from build123d import *

# Parameters (mm, degrees)
AUFSATZ_LINEAR_AUSTRAGEN1_DEPTH  = 16.09
WANDUNG2_T                       = -0.6
VERRUNDUNG1_R                    = 2
VERRUNDUNG2_R                    = 2
SKIZZE7_R                        = 2.5
AUFSATZ_LINEAR_AUSTRAGEN4_DEPTH  = 10
FASE3_SIZE                       = 0.5
AUFSATZ_LINEAR_AUSTRAGEN8_DEPTH  = 7.85
SKIZZE14_W                       = 3.695
SKIZZE14_H                       = 14.25
AUFSATZ_LINEAR_AUSTRAGEN9_DEPTH  = 2.94
SKIZZE15_W                       = 14.89
SKIZZE15_H                       = 14.52
AUFSATZ_LINEAR_AUSTRAGEN10_DEPTH = 1.06
SCHNITT_LINEAR_AUSTRAGEN1_REACH  = 12.16
SKIZZE16_W                       = 4.8
SKIZZE16_H                       = 5.3
SKIZZE17_W                       = 14.89
SKIZZE17_H                       = 14.52
AUFSATZ_LINEAR_AUSTRAGEN11_DEPTH = 1.06
SCHNITT_LINEAR_AUSTRAGEN2_REACH  = 12.16
SKIZZE18_W                       = 4.8
SKIZZE18_H                       = 5.3


with BuildPart() as part:
    # Skizze4 → Aufsatz-Linear austragen1 (new body)
    with BuildSketch(Plane.XY):
        Polygon((-6.4, 0), (-20, 14.7), (20, 14.7), (6.4, 0), align=None)
    extrude(amount=AUFSATZ_LINEAR_AUSTRAGEN1_DEPTH)

    # Wandung2
    wandung2_openings = [part.faces().sort_by_distance(p)[0] for p in [
        (0, 14.7, 8.045),
        (0, 0, 8.045),
    ]]
    offset(amount=WANDUNG2_T, openings=wandung2_openings, kind=Kind.INTERSECTION)

    # Verrundung1
    verrundung1_edges = [part.edges().sort_by_distance(p)[0] for p in [
        (12.382602743, 7.35, 15.49),
        (-12.382602743, 7.35, 15.49),
    ]]
    fillet(verrundung1_edges, radius=VERRUNDUNG1_R)

    # Verrundung2
    verrundung2_edges = [part.edges().sort_by_distance(p)[0] for p in [
        (12.382602743, 7.35, 0.6),
        (-12.382602743, 7.35, 0.6),
    ]]
    fillet(verrundung2_edges, radius=VERRUNDUNG2_R)

    # Skizze7 → Aufsatz-Linear austragen4 (add)
    with BuildSketch(Plane(origin=(0, 0, 0), x_dir=(-1, 0, 0), z_dir=(0, 0, -1))):
        with Locations((-14.281252926, 12.2)):
            Circle(SKIZZE7_R)
        with Locations((14.281252926, 12.2)):
            Circle(SKIZZE7_R)
    extrude(amount=AUFSATZ_LINEAR_AUSTRAGEN4_DEPTH)

    # Fase3
    fase3_edges = [part.edges().sort_by_distance(p)[0] for p in [
        (16.781252926, 12.2, -10),
        (-11.781252926, 12.2, -10),
    ]]
    chamfer(fase3_edges, length=FASE3_SIZE)

    # Skizze12 → Aufsatz-Linear austragen8 (add, symmetric)
    with BuildSketch(Plane.XY.offset(8.045)):
        Polygon((6.9, 0.540441176), (6.9, 10), (10.9, 10), (10.9, 4.863970588), align=None)
    aufsatz_linear_austragen8 = extrude(amount=AUFSATZ_LINEAR_AUSTRAGEN8_DEPTH, both=True)

    # Spiegeln6: Aufsatz-Linear austragen8 across plane
    add(aufsatz_linear_austragen8.mirror(Plane(origin=(0, 0, 0), x_dir=(0, 0, 1), z_dir=(1, 0, 0))))

    # Skizze14 → Aufsatz-Linear austragen9 (add)
    with BuildSketch(Plane.ZY.offset(-9.84)):
        with Locations((2.4475, 17.125)):
            Rectangle(SKIZZE14_W, SKIZZE14_H)
        with Locations((13.6425, 17.125)):
            Rectangle(SKIZZE14_W, SKIZZE14_H)
    aufsatz_linear_austragen9 = extrude(amount=AUFSATZ_LINEAR_AUSTRAGEN9_DEPTH)

    # Skizze15 → Aufsatz-Linear austragen10 (add)
    with BuildSketch(Plane(origin=(9.84, 0, 0), x_dir=(0, 0, -1), z_dir=(1, 0, 0))):
        with Locations((-8.045, 16.99)):
            Rectangle(SKIZZE15_W, SKIZZE15_H)
    extrude(amount=AUFSATZ_LINEAR_AUSTRAGEN10_DEPTH)

    # Skizze16 → Schnitt-Linear austragen1 (cut, up to next)
    with BuildSketch(Plane.ZY.offset(-9.84), mode=Mode.PRIVATE) as schnitt_linear_austragen1_sk1:
        with Locations((7.345, 21.6)):
            Rectangle(SKIZZE16_W, SKIZZE16_H)
    schnitt_linear_austragen1_tool1 = extrude(schnitt_linear_austragen1_sk1.sketch, amount=-SCHNITT_LINEAR_AUSTRAGEN1_REACH, mode=Mode.PRIVATE) & part.part
    add(schnitt_linear_austragen1_tool1.solids().sort_by_distance((9.84, 21.6, 7.345))[0], mode=Mode.SUBTRACT)

    # Spiegeln9: Aufsatz-Linear austragen9 across plane
    add(aufsatz_linear_austragen9.mirror(Plane(origin=(0, 0, 0), x_dir=(0, 0, 1), z_dir=(1, 0, 0))))

    # Skizze17 → Aufsatz-Linear austragen11 (add)
    with BuildSketch(Plane.ZY.offset(9.84)):
        with Locations((8.045, 16.99)):
            Rectangle(SKIZZE17_W, SKIZZE17_H)
    extrude(amount=AUFSATZ_LINEAR_AUSTRAGEN11_DEPTH)

    # Skizze18 → Schnitt-Linear austragen2 (cut, up to next)
    with BuildSketch(Plane(origin=(-9.84, 0, 0), x_dir=(0, 0, -1), z_dir=(1, 0, 0)), mode=Mode.PRIVATE) as schnitt_linear_austragen2_sk1:
        with Locations((-8.745, 21.6)):
            Rectangle(SKIZZE18_W, SKIZZE18_H)
    schnitt_linear_austragen2_tool1 = extrude(schnitt_linear_austragen2_sk1.sketch, amount=-SCHNITT_LINEAR_AUSTRAGEN2_REACH, mode=Mode.PRIVATE) & part.part
    add(schnitt_linear_austragen2_tool1.solids().sort_by_distance((-9.84, 21.6, 8.745))[0], mode=Mode.SUBTRACT)


solid = part.part
Could you check a few things on this model? Use its own coordinates, in mm. A direction names the side the tool comes from. Give positions to 0.01 mm unless a question says otherwise; leave off trailing zeros. Order: outer loops, then holes, each group sorted by start corner. A loop starts at its lowest first (then second) coordinate and runs counter-clockwise, first axis right, second up. Notation, with made-up numbers: (-5.5, -22) - (47.5, -22) arc R8 cw to (47.5, -10) - close; hole circle Ø4 at (56.25, 87.25). An arc over 180 degrees is marked (long way). One line per question, with ' | ' between items. Start each with the question number.
Item 1: I need wall thicknesses on probe 1 along X at (y, z) = (14.25, 11.25); probe 2 along Z at (x, y) = (-12.5, 11.5); probe 3 along Z at (x, y) = (2.5, 7.75). Which ranges of each line are inside material? Lowest first, please. Write a range as [from, to].
Item 2: Thinking about a two-plate mould opening in Z: for faces 1 (the cylindrical face through (5.74, 1.45, 0.95)), 2 (the flat face through (-9, 19, 0.6)), 3 (the flat face through (0, 9, 16.09)), 4 (the flat face through (9, 24.25, 13)), which applies, pulls with the +Z half, pulls with the -Z half, needs draft (parallel to the pull), parting line crosses it, or undercut?
Item 3: I want a section at C-C on z = -3.5. Write out the boundary of the cut face in (x, y).
Item 4: I want a section at A-A on y = 22.25. Write out the boundary of the cut face in (x, z) (3 decimals).
Item 5: I'm going to push flat-ended pins straight in: pin 1 Ø2 at (x, z) = (-14, 2) entering from +Y; pin 2 Ø0.8 at (x, y) = (-10.5, 21.5) entering from -Z; pin 3 Ø3 at (x, y) = (-3.5, 15) entering from -Z. Where does each tip first touch, or does it pass through?
Item 6: For faces 5 (the cylindrical face through (14.7, 10.7, 1.2)), 6 (the cylindrical face through (-12.44, 13.89, -4.68)), 7 (the flat face through (10, 22, 4.945)), which set-ups out of +Z, -Z, +X, -X, +Y, -Y let a thin tool reach every point of the face, with its end or its side?
Item 7: I want a section at B-B on x = 0. Write out the boundary of the cut face in (y, z).
Item 8: I want a section at D-D on x = -9. Write out the boundary of the cut face in (y, z) (3 decimals), then the cut area to 3 significant figures.
Verdict:
1) probe 1: [-19.58, -18.77], [-10.9, -9.84], [9.84, 10.9], [18.77, 19.58] | probe 2: [-10, 0.6], [15.49, 16.09] | probe 3: [0, 0.6], [15.49, 16.09]
2) face 1: undercut | face 2: pulls with the -Z half | face 3: pulls with the +Z half | face 4: needs draft
3) outline: circle Ø5 at (-14.28, 12.2); circle Ø5 at (14.28, 12.2)
4) outline: (-10.9, 0.6) - (-6.9, 0.6) - (-6.9, 4.295) - (-9.84, 4.295) - (-9.84, 6.345) - (-10.9, 6.345) - close; (-10.9, 11.145) - (-9.84, 11.145) - (-9.84, 11.795) - (-6.9, 11.795) - (-6.9, 15.49) - (-10.9, 15.49) - close; (6.9, 0.6) - (10.9, 0.6) - (10.9, 4.945) - (9.84, 4.945) - (9.84, 4.295) - (6.9, 4.295) - close; (6.9, 11.795) - (9.84, 11.795) - (9.84, 9.745) - (10.9, 9.745) - (10.9, 15.49) - (6.9, 15.49) - close
5) pin 1: y = 10.59 | pin 2: z = 0.6 | pin 3: z = 0
6) face 5: +Y | face 6: -Z | face 7: +X, +Y
7) outline: (0, 0) - (14.7, 0) - (14.7, 0.6) - (0, 0.6) - close; (0, 15.49) - (14.7, 15.49) - (14.7, 16.09) - (0, 16.09) - close
8) outline: (2.81, 0) - (14.7, 0) - (14.7, 0.6) - (24.25, 0.6) - (24.25, 4.295) - (10, 4.295) - (10, 11.795) - (24.25, 11.795) - (24.25, 15.49) - (14.7, 15.49) - (14.7, 16.09) - (2.81, 16.09) - close | area: 227 mm^2
